The drawing under review shows one solid part. Ordinate dimensions are in mm from its lowest x, y, z. A direction names the side the tool comes from. Coordinates: 2 decimals unless noted, no trailing zeros. Order: outer loops, then holes, each group sorted by start corner. A loop starts at its lowest first (then second) coordinate and runs counter-clockwise, first axis right, second up.
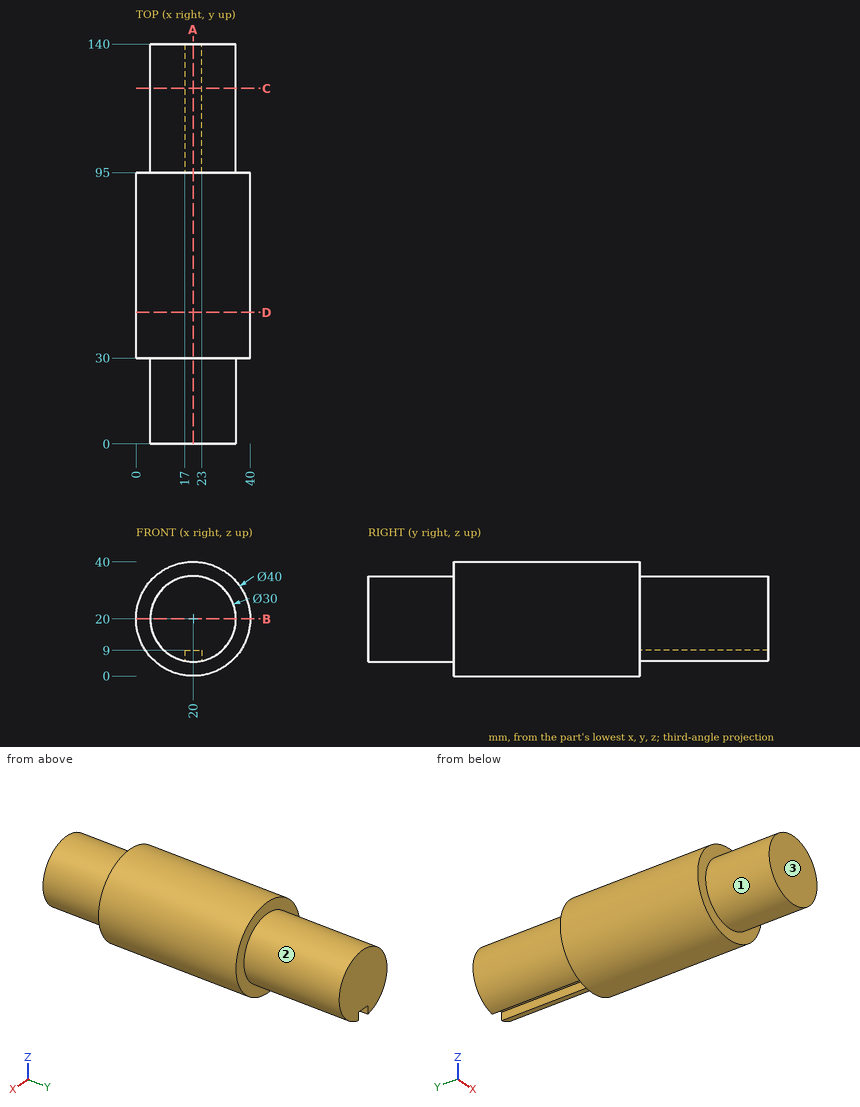
1. Add section C-C (y = 124.5). Give the boundary of the cut face in (x, z), and give its area (3 significant figures).
2. Insertion check: pin 1 (8 mm diameter, centred on y = 88.5, z = 35.5, fed in from -X); pin 2 (2 mm diameter, centred on y = 42, z = 22.5, fed in from -X); pin 3 (1 mm diameter, centred on y = 14.5, z = 30, fed in from -X). Each pin has a flat end and moves straight along its axis. Give the tip position at first contact, or say it passes through.
3. To check wall thickness, follow line 1 (Y direction, x = 38.5, z = 19.5); line 2 (Y direction, x = 19.5, z = 8.5); line 3 (Z direction, x = 13, y = 60) (3 decimals). State the ranges of each line that lie inside material, in increasing order.
4. Add section B-B (z = 20). Give the boundary of the cut face in (x, y).
5. For the marked faces 1, 2 and 3, list the 3-axis set-ups (+Z, -Z, +X, -X, +Y, -Y) from which the entire face can be reached by the end or side of a thin tool; tool diameter is ignored.
6. Add section D-D (y = 46). Give the boundary of the cut face in (x, z).
7. Add section A-A (x = 20). Give the boundary of the cut face in (y, z).
Solution:
1. outline: (17, 5.3) - (17, 9) - (23, 9) - (23, 5.3) arc R15 ccw (long way) to start
1. area: 683 mm2
2. pin 1: stops at x = 3.64
2. pin 2: stops at x = 0.06
2. pin 3: stops at x = 8.39
3. line 1: y = 30 to 95
3. line 2: y = 0 to 95
3. line 3: z = 1.265 to 38.735
4. outline: (0, 30) - (5, 30) - (5, 0) - (35, 0) - (35, 30) - (40, 30) - (40, 95) - (35, 95) - (35, 140) - (5, 140) - (5, 95) - (0, 95) - close
5. face 1: -Y
5. face 2: +Y
5. face 3: +Z, -Z, +X, -X, -Y
6. outline: circle Ø40 at (20, 20)
7. outline: (0, 5) - (30, 5) - (30, 0) - (95, 0) - (95, 9) - (140, 9) - (140, 35) - (95, 35) - (95, 40) - (30, 40) - (30, 35) - (0, 35) - close
